Design review of the part built by this model. Coordinates are the model's own, in mm. A direction names the side the tool comes from. Coordinates: 2 decimals unless noted, no trailing zeros. Write each loop counter-clockwise with the first axis right and the second up, starting at its lowest first coordinate (ties: lowest second). Pieces come first, ordered by that corner, then holes. Notation, with made-up numbers: (87, 1.25) - (125, 1.25) arc R32 ccw to (125, 34.25) - close; hole circle Ø2 at (-26, 69.5). An arc over 180 degrees is marked (long way). Answer as CSV lines item,"result". Start each with the question number.
Q1. Machinability: for faces 4 (the face through (80, 0.4, 304.8)), 5 (the face through (-175, 73, 301.625)), 6 (the face through (-280, -25, -304.8)), which of the approach directions +Z, -Z, +X, -X, +Y, -Y give a long, thin tool a straight path to every point of the face, cutting with its end or side? Answer none if there is none.
Q2. For line 1 along Z through (x, y) = (48.5, 7); line 2 along Y through (x, z) = (177.8, 34.5) (1 decimal); line 3 along X through (y, z) = (6, 57), list the stretches that pass through material, from the lowest coordinate up. Write a range as [from, to].
Q3. Mouldability with a two-part tool opening along Y and no side actions: class faces 1 (the face through (322, 1.588, 175)), 2 (the face through (-222, 60, -290.512)), 3 (the face through (145.41, -34.264, -298.361)) as pulls with the +Y half, pulls with the -Y half, needs draft (parallel to the pull), parting line crosses it, or undercut.
Q4. Clearance check with flat-ended pins moving along their axes: pin 1 (10 mm diameter, centred on y = -8.5, z = 301.5, fed in from +X); pin 2 (4 mm diameter, centred on y = 97, z = -299.5, fed in from +X); pin 3 (9 mm diameter, centred on x = 78.5, y = 138.5, fed in from -Z). State where each tip first meets the part, or that it passes through.
Q5. We need section B-B (z = -12). State how many separate pieces and enclosed holes the cut face has, plus the area to 3 significant figures.
Q6. We need section A-A (x = -54). Write out the cut boundary in (y, z) (1 decimal), plus the area to 3 significant figures.
from build123d import *

# Parameters (mm, degrees)
BOSS_EXTRUDE4_DEPTH  = 144.4625
BOSS_EXTRUDE5_REACH  = 709.466
BOSS_EXTRUDE6_START  = 304.8
SKETCH8_R            = 7.9375
BOSS_EXTRUDE6_DEPTH  = 12.7
BOSS_EXTRUDE11_START = -12.7
SKETCH11_R           = 7.9375
BOSS_EXTRUDE11_DEPTH = 12.7
BOSS_EXTRUDE12_REACH = 521.326
BOSS_EXTRUDE15_START = -12.7
SKETCH13_R           = 7.9375
BOSS_EXTRUDE15_DEPTH = 12.7
SKETCH14_R           = 7.9375
BOSS_EXTRUDE16_DEPTH = 12.7
SKETCH15_W           = 38.1
SKETCH15_H           = 1.5875
BOSS_EXTRUDE17_DEPTH = 63.5
CUT_EXTRUDE1_REACH   = 712.196
SKETCH18_W           = 304.8
SKETCH18_H           = 12.7
BOSS_EXTRUDE21_DEPTH = 1.5875
BOSS_EXTRUDE23_DEPTH = 12.7


with BuildPart() as part:
    # Sweep1: sweep along a path in Sketch1
    with BuildLine(Plane(origin=(0, 0, 0), x_dir=(1, 0, 0), z_dir=(0, 1, 0))) as sweep1_path:
        Line((-330.2, -304.8), (330.2, -304.8))
        Line((330.2, -304.8), (330.2, 304.8))
        Line((330.2, 304.8), (-330.2, 304.8))
        Line((-330.2, 304.8), (-330.2, -304.8))
    # Sketch2 → Sweep1 (sweep)
    with BuildSketch(Plane(origin=(0, 0, 0), x_dir=(0, 0, -1), z_dir=(1, 0, 0))):
        Polygon((-304.8, 0), (-292.1, 0), (-292.1, 1.5875), (-303.2125, 1.5875), (-303.2125, 12.7), (-304.8, 12.7), align=None)
    sweep(path=sweep1_path.line, transition=Transition.RIGHT)



with BuildPart() as body_2:
    # Sweep2: sweep along a path in Sketch4
    with BuildLine(Plane(origin=(0, 147.6375, 0), x_dir=(1, 0, 0), z_dir=(0, 1, 0))) as sweep2_path:
        Line((-330.2, -304.8), (330.2, -304.8))
        Line((330.2, -304.8), (330.2, 304.8))
        Line((330.2, 304.8), (-330.2, 304.8))
        Line((-330.2, 304.8), (-330.2, -304.8))
    # Sketch5 → Sweep2 (sweep)
    with BuildSketch(Plane(origin=(0, 0, 0), x_dir=(0, 0, -1), z_dir=(1, 0, 0))):
        Polygon((304.8, 147.6375), (304.8, 134.9375), (303.2125, 134.9375), (303.2125, 146.05), (292.1, 146.05), (292.1, 147.6375), align=None)
    sweep(path=sweep2_path.line, transition=Transition.RIGHT)


with BuildPart() as part_1:
    add(part.part)

    add(body_2.part)  # Boss-Extrude4 merges body 2
    # Sketch6 → Boss-Extrude4 (add)
    with BuildSketch(Plane(origin=(0, 1.5875, 0), x_dir=(1, 0, 0), z_dir=(0, 1, 0))):
        Polygon((315.9125, -303.2125), (328.6125, -303.2125), (328.6125, -290.5125), (327.025, -290.5125), (327.025, -301.625), (315.9125, -301.625), align=None)
        Polygon((12.7, -303.2125), (12.7, -301.625), (1.5875, -301.625), (1.5875, -290.5125), (0, -290.5125), (0, -303.2125), align=None)
    boss_extrude4 = extrude(amount=BOSS_EXTRUDE4_DEPTH)

    # Mirror1: Boss-Extrude4 across plane
    add(boss_extrude4.mirror(Plane.XY))

    # Boss-Extrude5: up to this face of the body (flat: up to its plane)
    boss_extrude5_end = Plane(part_1.part.faces().sort_by_distance((-164.30625, 140.49375, -303.2125))[0])
    # Sketch7 → Boss-Extrude5 (add, up to the picked face)
    with BuildSketch(Plane(origin=(0, 0, 303.2125), x_dir=(-1, 0, 0), z_dir=(0, 0, -1)), mode=Mode.PRIVATE) as boss_extrude5_sk1:
        Polygon((-238.125, 146.05), (-238.125, 133.35), (-236.5375, 133.35), (-236.5375, 144.4625), (-225.425, 144.4625), (-225.425, 146.05), align=None)
    boss_extrude5_tool1 = split(extrude(boss_extrude5_sk1.sketch, amount=BOSS_EXTRUDE5_REACH, mode=Mode.PRIVATE), bisect_by=boss_extrude5_end, keep=Keep.BOTH, mode=Mode.PRIVATE)
    # Sketch7 → Boss-Extrude5 (add, up to the picked face)
    with BuildSketch(Plane(origin=(0, 0, 303.2125), x_dir=(-1, 0, 0), z_dir=(0, 0, -1)), mode=Mode.PRIVATE) as boss_extrude5_sk2:
        Polygon((-130.175, 146.05), (-117.475, 146.05), (-117.475, 133.35), (-119.0625, 133.35), (-119.0625, 144.4625), (-130.175, 144.4625), align=None)
    boss_extrude5_tool2 = split(extrude(boss_extrude5_sk2.sketch, amount=BOSS_EXTRUDE5_REACH, mode=Mode.PRIVATE), bisect_by=boss_extrude5_end, keep=Keep.BOTH, mode=Mode.PRIVATE)
    # Sketch7 → Boss-Extrude5 (add, up to the picked face)
    with BuildSketch(Plane(origin=(0, 0, 303.2125), x_dir=(-1, 0, 0), z_dir=(0, 0, -1)), mode=Mode.PRIVATE) as boss_extrude5_sk3:
        Polygon((-76.2, 0), (-76.2, -1.5875), (-65.0875, -1.5875), (-65.0875, -12.7), (-63.5, -12.7), (-63.5, 0), align=None)
    boss_extrude5_tool3 = split(extrude(boss_extrude5_sk3.sketch, amount=BOSS_EXTRUDE5_REACH, mode=Mode.PRIVATE), bisect_by=boss_extrude5_end, keep=Keep.BOTH, mode=Mode.PRIVATE)
    add(boss_extrude5_tool1.solids().sort_by(Axis((237.945395, 139.7, 303.2125), (0, 0, -1)))[0])
    add(boss_extrude5_tool2.solids().sort_by(Axis((123.825, 145.870395, 303.2125), (0, 0, -1)))[0])
    add(boss_extrude5_tool3.solids().sort_by(Axis((76.020395, -0.79375, 303.2125), (0, 0, -1)))[0])

    # Sketch8 → Boss-Extrude6 (add)
    with BuildSketch(Plane.XY.offset(BOSS_EXTRUDE6_START)):
        with BuildLine():
            Line((127, -12.7), (127, 0))
            Line((127, 0), (228.6, 0))
            Line((228.6, 0), (228.6, -12.7))
            Line((228.6, -12.7), (192.288023852, -55.23180333))
            ThreePointArc((192.288023852, -55.23180333), (177.8, -61.9125), (163.311976148, -55.23180333))
            Line((163.311976148, -55.23180333), (127, -12.7))
        make_face()
        with Locations((177.8, -42.8625)):
            Circle(SKETCH8_R, mode=Mode.SUBTRACT)
    extrude(amount=-BOSS_EXTRUDE6_DEPTH)

    # Sketch11 → Boss-Extrude11 (add)
    with BuildSketch(Plane(origin=(0, 0, -304.8), x_dir=(-1, 0, 0), z_dir=(0, 0, -1)).offset(BOSS_EXTRUDE11_START)):
        with BuildLine():
            Line((-127, -12.7), (-127, 0))
            Line((-127, 0), (-228.6, 0))
            Line((-228.6, 0), (-228.6, -12.7))
            Line((-228.6, -12.7), (-192.288023852, -55.23180333))
            ThreePointArc((-192.288023852, -55.23180333), (-177.8, -61.9125), (-163.311976148, -55.23180333))
            Line((-163.311976148, -55.23180333), (-127, -12.7))
        make_face()
        with Locations(Location((-177.8, -42.8625, 0), (0, 0, 180))):
            Circle(SKETCH11_R, mode=Mode.SUBTRACT)
    extrude(amount=BOSS_EXTRUDE11_DEPTH)

    # Boss-Extrude12: up to this face of the body (flat: up to its plane)
    boss_extrude12_end = Plane(part_1.part.faces().sort_by_distance((328.6125, 7.14375, 0))[0])
    # Sketch12 → Boss-Extrude12 (add, up to the picked face)
    with BuildSketch(Plane.ZY.offset(-63.5), mode=Mode.PRIVATE) as boss_extrude12_sk1:
        Polygon((-25.4, 0), (-25.4, 12.7), (-26.9875, 12.7), (-26.9875, 1.5875), (-38.1, 1.5875), (-38.1, 0), align=None)
    boss_extrude12_tool1 = split(extrude(boss_extrude12_sk1.sketch, amount=-BOSS_EXTRUDE12_REACH, mode=Mode.PRIVATE), bisect_by=boss_extrude12_end, keep=Keep.BOTH, mode=Mode.PRIVATE)
    # Sketch12 → Boss-Extrude12 (add, up to the picked face)
    with BuildSketch(Plane.ZY.offset(-63.5), mode=Mode.PRIVATE) as boss_extrude12_sk2:
        Polygon((25.4, 0), (25.4, 12.7), (26.9875, 12.7), (26.9875, 1.5875), (38.1, 1.5875), (38.1, 0), align=None)
    boss_extrude12_tool2 = split(extrude(boss_extrude12_sk2.sketch, amount=-BOSS_EXTRUDE12_REACH, mode=Mode.PRIVATE), bisect_by=boss_extrude12_end, keep=Keep.BOTH, mode=Mode.PRIVATE)
    add(boss_extrude12_tool1.solids().sort_by(Axis((63.5, 6.35, -25.579605), (1, 0, 0)))[0])
    add(boss_extrude12_tool2.solids().sort_by(Axis((63.5, 6.35, 25.579605), (1, 0, 0)))[0])

    # Sketch13 → Boss-Extrude15 (add)
    with BuildSketch(Plane(origin=(0, 0, -38.1), x_dir=(-1, 0, 0), z_dir=(0, 0, -1)).offset(BOSS_EXTRUDE15_START)):
        with BuildLine():
            Line((-127, 0), (-228.6, 0))
            Line((-228.6, 0), (-228.6, -12.7))
            Line((-228.6, -12.7), (-192.288023852, -55.23180333))
            ThreePointArc((-192.288023852, -55.23180333), (-177.8, -61.9125), (-163.311976148, -55.23180333))
            Line((-163.311976148, -55.23180333), (-127, -12.7))
            Line((-127, -12.7), (-127, 0))
        make_face()
        with Locations(Location((-177.8, -42.8625, 0), (0, 0, 180))):
            Circle(SKETCH13_R, mode=Mode.SUBTRACT)
    extrude(amount=BOSS_EXTRUDE15_DEPTH)

    # Sketch14 → Boss-Extrude16 (add)
    with BuildSketch(Plane.XY.offset(38.1)):
        with BuildLine():
            Line((228.6, -12.7), (228.6, 0))
            Line((228.6, 0), (127, 0))
            Line((127, 0), (127, -12.7))
            Line((127, -12.7), (163.311976148, -55.23180333))
            ThreePointArc((163.311976148, -55.23180333), (177.8, -61.9125), (192.288023852, -55.23180333))
            Line((192.288023852, -55.23180333), (228.6, -12.7))
        make_face()
        with Locations((177.8, -42.8625)):
            Circle(SKETCH14_R, mode=Mode.SUBTRACT)
    extrude(amount=-BOSS_EXTRUDE16_DEPTH)

    # Sketch15 → Boss-Extrude17 (add)
    with BuildSketch(Plane(origin=(0, 12.7, 0), x_dir=(1, 0, 0), z_dir=(0, 1, 0))):
        with Locations((-279.4, 305.59375)):
            Rectangle(SKETCH15_W, SKETCH15_H)
        with Locations((-279.4, -305.59375)):
            Rectangle(SKETCH15_W, SKETCH15_H)
    extrude(amount=-BOSS_EXTRUDE17_DEPTH)

    # Cut-Extrude1: up to this face of the body (flat: up to its plane)
    cut_extrude1_end = Plane(part_1.part.faces().sort_by_distance((0, 141.2875, 304.8))[0])
    # Sketch18 → Cut-Extrude1 (cut, up to the picked face)
    with BuildSketch(Plane(origin=(0, 0, -304.8), x_dir=(-1, 0, 0), z_dir=(0, 0, -1)), mode=Mode.PRIVATE) as cut_extrude1_sk1:
        with Locations((177.8, 141.2875)):
            Rectangle(SKETCH18_W, SKETCH18_H)
    cut_extrude1_tool1 = split(extrude(cut_extrude1_sk1.sketch, amount=-CUT_EXTRUDE1_REACH, mode=Mode.PRIVATE), bisect_by=cut_extrude1_end, keep=Keep.BOTH, mode=Mode.PRIVATE)
    add(cut_extrude1_tool1.solids().sort_by(Axis((-177.8, 141.2875, -304.8), (0, 0, 1)))[0], mode=Mode.SUBTRACT)

    # Sketch19 → Boss-Extrude21 (add)
    with BuildSketch(Plane.XY.offset(-303.2125)):
        Polygon((-25.4, 144.78), (-328.6125, 14.526382188), (-323.599797289, 2.8575), (-20.387297289, 133.111117812), align=None)
    boss_extrude21 = extrude(amount=BOSS_EXTRUDE21_DEPTH)

    # Sketch20 → Boss-Extrude23 (add)
    with BuildSketch(Plane(origin=(0, 0, -303.2125), x_dir=(-1, 0, 0), z_dir=(0, 0, -1))):
        Polygon((25.4, 144.78), (328.6125, 14.526382188), (327.985912161, 13.067771915), (24.773412161, 143.321389726), align=None)
    boss_extrude23 = extrude(amount=-BOSS_EXTRUDE23_DEPTH)

    # Mirror2: Boss-Extrude21, Boss-Extrude23 across plane
    add(boss_extrude21.mirror(Plane.XY))
    add(boss_extrude23.mirror(Plane.XY))


solid = part_1.part
Results list:
1,face 4,"+Z, +X, +Y, -Y"
1,face 5,"none"
1,face 6,"-X, -Y"
2,line 1,"z = [-304.8, -303.21], [303.21, 304.8]"
2,line 2,"y = [-61.9, -50.8], [-34.9, 1.6]"
2,line 3,"x = [-330.2, -328.61], [328.61, 330.2]"
3,face 1,"undercut"
3,face 2,"needs draft"
3,face 3,"pulls with the -Y half"
4,pin 1,"stops at x = 228.6"
4,pin 2,"stops at x = 328.61"
4,pin 3,"stops at z = -304.8"
5,separate pieces,"6"
5,enclosed holes,"0"
5,area,"227 mm2"
6,outline,"(0, -304.8) - (12.7, -304.8) - (12.7, -303.2) - (1.6, -303.2) - (1.6, -292.1) - (0, -292.1) - close; (0, 292.1) - (1.6, 292.1) - (1.6, 303.2) - (12.7, 303.2) - (12.7, 304.8) - (0, 304.8) - close; (118.7, -303.2) - (132.5, -303.2) - (132.5, -290.5) - (130.8, -290.5) - (130.8, -301.6) - (118.7, -301.6) - close; (118.7, 301.6) - (130.8, 301.6) - (130.8, 290.5) - (132.5, 290.5) - (132.5, 303.2) - (118.7, 303.2) - close"
6,area,"158 mm2"
